Geometry: final body of the model. Coordinates: model frame, mm. A direction names the side the tool comes from. Coordinates: 2 decimals unless noted, no trailing zeros. Loops run counter-clockwise (first coordinate to the right, second up) from the corner with the lowest first, then second, coordinate; pieces in that order, holes last. Notation, with made-up numbers: (63.25, 35) - (111.25, 35) arc R28 cw to (111.25, 71) - close; hole circle Ø5 at (-36, 84.5). An arc over 180 degrees is marked (long way). Answer in a Markdown table with one row per item.
from build123d import *

# Parameters (mm, degrees)
SKETCH1_W           = 280
SKETCH1_H           = 200
SKETCH1_R           = 5
SKETCH1_R_2         = 6
BOSS_EXTRUDE1_DEPTH = 30
SKETCH2_R           = 7
CUT_EXTRUDE1_DEPTH  = 30
BOSS_EXTRUDE3_START = -10
SKETCH3_R           = 5
BOSS_EXTRUDE3_DEPTH = 10
SKETCH4_R           = 6
CUT_EXTRUDE2_DEPTH  = 30
SKETCH5_R           = 4
CUT_EXTRUDE3_DEPTH  = 200
SKETCH6_R           = 2.108291455
SKETCH6_R_2         = 2.313215084
CUT_EXTRUDE7_DEPTH  = 0.6


with BuildPart() as part:
    # Sketch1 → Boss-Extrude1 (new body)
    with BuildSketch(Plane.XY):
        Rectangle(SKETCH1_W, SKETCH1_H)
        with Locations((-120, -85)):
            Circle(SKETCH1_R, mode=Mode.SUBTRACT)
        with Locations((120, -85)):
            Circle(SKETCH1_R, mode=Mode.SUBTRACT)
        with Locations((-65, -85)):
            Circle(SKETCH1_R, mode=Mode.SUBTRACT)
        with Locations((65, -85)):
            Circle(SKETCH1_R, mode=Mode.SUBTRACT)
        with Locations((65, 85)):
            Circle(SKETCH1_R, mode=Mode.SUBTRACT)
        with Locations((-65, 85)):
            Circle(SKETCH1_R, mode=Mode.SUBTRACT)
        with Locations((-120, 85)):
            Circle(SKETCH1_R, mode=Mode.SUBTRACT)
        with Locations((120, 85)):
            Circle(SKETCH1_R, mode=Mode.SUBTRACT)
        Circle(SKETCH1_R_2, mode=Mode.SUBTRACT)
    extrude(amount=BOSS_EXTRUDE1_DEPTH)

    # Sketch2 → Cut-Extrude1 (cut)
    with BuildSketch(Plane(origin=(0, 0, 0), x_dir=(-1, 0, 0), z_dir=(0, 0, -1))):
        with Locations((-120, 85)):
            Circle(SKETCH2_R)
        with Locations((120, 85)):
            Circle(SKETCH2_R)
        with Locations((65, -85)):
            Circle(SKETCH2_R)
        with Locations((-65, -85)):
            Circle(SKETCH2_R)
    extrude(amount=-CUT_EXTRUDE1_DEPTH, mode=Mode.SUBTRACT)

    # Sketch3 → Boss-Extrude3 (add)
    with BuildSketch(Plane.XY.offset(30).offset(BOSS_EXTRUDE3_START)):
        with Locations((-120, -85)):
            Circle(SKETCH3_R)
        with Locations((120, -85)):
            Circle(SKETCH3_R)
        with Locations((-65, 85)):
            Circle(SKETCH3_R)
        with Locations((65, 85)):
            Circle(SKETCH3_R)
    extrude(amount=BOSS_EXTRUDE3_DEPTH)

    # Sketch4 → Cut-Extrude2 (cut)
    with BuildSketch(Plane.XY.offset(30)):
        with Locations((-102, -82)):
            Circle(SKETCH4_R)
        with Locations(Location((102, -82, 0), (0, 0, 180))):
            Circle(SKETCH4_R)
    extrude(amount=-CUT_EXTRUDE2_DEPTH, mode=Mode.SUBTRACT)

    # Sketch5 → Cut-Extrude3 (cut)
    with BuildSketch(Plane(origin=(0, -100, 0), x_dir=(-1, 0, 0), z_dir=(0, -1, 0))):
        with Locations(Location((40, -15, 0), (0, 0, 180))):
            Circle(SKETCH5_R)
        with Locations((-40, -15)):
            Circle(SKETCH5_R)
    extrude(amount=-CUT_EXTRUDE3_DEPTH, mode=Mode.SUBTRACT)

    # Sketch6 → Cut-Extrude7 (cut)
    # profile 1 of 6: a face of its own
    with BuildSketch(Plane.XY):
        with BuildLine():
            Line((-11.104324014, 17.945069254), (-10.223815884, 17.945042681))
            ThreePointArc((-10.223815884, 17.945042681), (-5.282103106, 15.803086541), (-7.097802531, 20.873760745))
            ThreePointArc((-7.097802531, 20.873760745), (-10.28034524, 23.758493076), (-7.293051975, 26.844969654))
            Line((-7.293051975, 26.844969654), (-4.090157048, 26.844872994))
            Line((-4.090157048, 26.844872994), (-4.090183621, 25.964364865))
            Line((-4.090183621, 25.964364865), (-5.174581416, 25.964397591))
            ThreePointArc((-5.174581416, 25.964397591), (-4.318518193, 23.565420803), (-5.622908359, 21.377613643))
            ThreePointArc((-5.622908359, 21.377613643), (-5.263734666, 14.711153724), (-11.104324014, 17.945069254))
        make_face()
        with Locations((-7.293142173, 23.85617007)):
            Circle(SKETCH6_R, mode=Mode.SUBTRACT)
    # profile 2 of 6: a face of its own
    with BuildSketch(Plane.XY):
        Polygon((1.840305593, 22.213875796), (2.720813722, 22.213849223), (2.720631568, 16.17802246), (1.840123439, 16.178049033), align=None)
    # profile 3 of 6: a face of its own
    with BuildSketch(Plane.XY):
        Polygon((-1.577208157, 16.178152164), (-0.696700027, 16.178125591), (-0.696381672, 26.727084122), (-1.576889802, 26.727110694), align=None)
    # profile 4 of 6: a face of its own
    with BuildSketch(Plane.XY):
        with BuildLine():
            Line((9.865957526, 20.914655791), (9.865984634, 21.812912632))
            Line((9.865984634, 21.812912632), (10.746492764, 21.81288606))
            Line((10.746492764, 21.81288606), (10.599564257, 15.942836291))
            Line((10.599564257, 15.942836291), (9.865807483, 15.942858434))
            Line((9.865807483, 15.942858434), (9.865834591, 16.841115276))
            ThreePointArc((9.865834591, 16.841115276), (4.212206408, 18.878056155), (9.865957526, 20.914655791))
        make_face()
        with Locations((7.40592962, 18.877959772)):
            Circle(SKETCH6_R_2, mode=Mode.SUBTRACT)
    # profile 5 of 6: a face of its own
    with BuildSketch(Plane.XY):
        Polygon((1.84041394, 25.804070666), (1.840441794, 26.727007563), (10.746641058, 26.726738785), (10.746613205, 25.803801888), align=None)
    # profile 6 of 6: a face of its own
    with BuildSketch(Plane.XY):
        Polygon((1.840341861, 23.415664961), (10.746541125, 23.415396183), (10.746567668, 24.294913294), (1.840368404, 24.295182072), align=None)
    extrude(amount=CUT_EXTRUDE7_DEPTH, mode=Mode.SUBTRACT)


solid = part.part
(1) Access query for faces 1 (the face through (65.91, -78.06, 14.79)), 2 (the face through (-115.381, -86.915, 9.86)). Directions: +Z, -Z, +X, -X, +Y, -Y. A direction counts if a zero-diameter tool reaches every point of the face in a straight line with its end or side. Return the directions, or none.
Verdict:
| item | result |
|---|---|
| face 1 | +Z, -Z |
| face 2 | -Z |
(2) Cut plane B-B on z = 5.5. State how many separate pieces and enclosed holes the cut face has, then the cut area to 3 significant figures.
Verdict:
| item | result |
|---|---|
| separate pieces | 1 |
| enclosed holes | 11 |
| area | 54,700 mm² |
(3) Cut plane D-D on z = 24.25. Output: boundary loops of the cut face in (x, y).
Verdict:
| item | result |
|---|---|
| outline | (-140, -100) - (140, -100) - (140, 100) - (-140, 100) - close; hole circle Ø14 at (-120, 85); hole circle Ø12 at (-102, -82); hole circle Ø14 at (-65, -85); hole circle Ø12 at (0, 0); hole circle Ø14 at (65, -85); hole circle Ø12 at (102, -82); hole circle Ø14 at (120, 85) |
(4) First-contact query: pin 1 Ø9 at (x, y) = (65, 85) entering from -Z. Flat tip, straight axial feed; report the tip coordinate or a pass-through.
Verdict:
| item | result |
|---|---|
| pin 1 | stops at z = 20 |
(5) Pull-direction query (X, two-part tool) for faces 3 (the face through (-42.95, -1.4, 17.7)), 4 (the face through (-2, 24, 0)), 5 (the face through (140, -1, 15)); classes: pulls with the +X half, pulls with the -X half, needs draft (parallel to the pull), parting line crosses it, or undercut.
Verdict:
| item | result |
|---|---|
| face 3 | undercut |
| face 4 | needs draft |
| face 5 | pulls with the +X half |
(6) Cut plane A-A on x = 65. Output: boundary loops of the cut face in (y, z), then the cut area to 3 significant figures.
Verdict:
| item | result |
|---|---|
| outline | (-100, 0) - (-92, 0) - (-92, 30) - (-100, 30) - close; (-78, 0) - (80, 0) - (80, 20) - (90, 20) - (90, 0) - (100, 0) - (100, 30) - (-78, 30) - close |
| area | 5,380 mm² |
(7) Ray query, probe 1 along Y at (x, z) = (-65, 15.75); probe 2 along X at (y, z) = (-40, 11.75); probe 3 along X at (y, z) = (1, 16.25). Return the intervals inside material, ascending.
Verdict:
| item | result |
|---|---|
| probe 1 | y = -100 to -92, -78 to 80, 90 to 100 |
| probe 2 | x = -140 to -42.33, -37.67 to 37.67, 42.33 to 140 |
| probe 3 | x = -140 to -43.8, -36.2 to -5.92, 5.92 to 36.2, 43.8 to 140 |
